```python
from build123d import *

# Parameters (mm, degrees)
EXTRUDE1_DEPTH = 25.146
HOLE1_D        = 16.002
HOLE1_DEPTH    = 2.286
CHAMFER1_SIZE  = 0.254
CHAMFER2_SIZE  = 0.762
CHAMFER3_SIZE  = 0.762
CHAMFER4_SIZE  = 0.762


with BuildPart() as part:
    # Sketch1 → Extrude1 (new body)
    with BuildSketch(Plane(origin=(0, 0, 0), x_dir=(0, -1, 0), z_dir=(-1, 0, 0))):
        Polygon((31.75, 18.330871047), (0, 36.661742094), (-31.75, 18.330871047), (-31.75, -18.330871047), (0, -36.661742094), (31.75, -18.330871047), align=None)
    extrude(amount=-EXTRUDE1_DEPTH)

    # Sketch2 → Cut-Revolve1 (revolve, cut)
    with BuildSketch(Plane.XY, mode=Mode.PRIVATE) as cut_revolve1_sk:
        with BuildLine():
            Line((0, 27.8003), (0, 0))
            Line((0, 0), (25.146, 0))
            Line((25.146, 0), (25.146, 10.4775))
            Line((25.146, 10.4775), (24.892, 10.4775))
            Line((24.892, 10.4775), (24.892, 6.1849))
            Line((24.892, 6.1849), (22.3393, 5.642306865))
            Line((22.3393, 5.642306865), (21.675393135, 4.9784))
            Line((21.675393135, 4.9784), (14.986, 4.9784))
            Line((14.986, 4.9784), (14.986, 27.4955))
            Line((14.986, 27.4955), (12.7, 27.4955))
            ThreePointArc((12.7, 27.4955), (12.512653369, 27.717323293), (12.234410309, 27.8003))
            Line((12.234410309, 27.8003), (0, 27.8003))
        make_face()
    revolve(cut_revolve1_sk.sketch.rotate(Axis((0, 0, 0), (1, 0, 0)), 270), axis=Axis((0, 0, 0), (1, 0, 0)), mode=Mode.SUBTRACT)  # turned: the seam where the file's is

    # Hole1
    with Locations(Plane.ZY.offset(-14.986)):
        with Locations((0, 15.24)):
            Hole(HOLE1_D / 2, depth=HOLE1_DEPTH)

    # Chamfer1
    chamfer1_edges = [part.edges().sort_by_distance(p)[0] for p in [
        (0, 0, 27.8003),
    ]]
    chamfer(chamfer1_edges, length=CHAMFER1_SIZE)

    # Chamfer2
    chamfer2_edges = [part.edges().sort_by_distance(p)[0] for p in [
        (14.986, 0, 4.9784),
    ]]
    chamfer(chamfer2_edges, length=CHAMFER2_SIZE)

    # Chamfer3
    chamfer3_edges = [part.edges().sort_by_distance(p)[0] for p in [
        (0, -15.875, -27.49630657),
        (0, 15.875, -27.49630657),
        (0, 31.75, 0),
        (0, 15.875, 27.49630657),
        (0, -15.875, 27.49630657),
        (0, -31.75, 0),
    ]]
    chamfer(chamfer3_edges, length=CHAMFER3_SIZE)

    # Chamfer4
    chamfer4_edges = [part.edges().sort_by_distance(p)[0] for p in [
        (25.146, 15.875, 27.49630657),
        (25.146, 31.75, 0),
        (25.146, 15.875, -27.49630657),
        (25.146, -15.875, -27.49630657),
        (25.146, -31.75, 0),
        (25.146, -15.875, 27.49630657),
    ]]
    chamfer(chamfer4_edges, length=CHAMFER4_SIZE)


solid = part.part
```
Read the model definition and answer for the solid it produces. Units are mm, in the model's axes. A direction names the side the tool comes from. Coordinates: 2 decimals unless noted, no trailing zeros. Write each loop counter-clockwise with the first axis right and the second up, starting at its lowest first coordinate (ties: lowest second). Pieces come first, ordered by that corner, then holes. Notation, with made-up numbers: (9.5, 87) - (46.5, 87) arc R13 ccw to (46.5, 92) - close; hole circle Ø5 at (48.25, -33.5). An arc over 180 degrees is marked (long way). Answer as a JSON object with one key per item and string values. Group by question number.
1. The mould has two halves that part along Y. Classify faces 4 (the flat face through (24.77, 15.46, 27.29)), 5 (the flat face through (0, 12, -26)), 6 (the flat face through (24.77, -15.46, -27.29)), 7 (the flat face through (14.986, -6, 6)): +Y half, -Y half, draft (parallel to the pull), parting line (faces both ways), or undercut.
2. Each of these flat-tipped pins is pushed along its axis until it touches: P1, Ø8, axis at y = -15.5, z = -17, coming from the -X side; P2, Ø4, axis at x = 5, y = -2.5, coming from the -Z side; P3, Ø1.5, axis at x = 7, z = 20, coming from the +Y side. Where does it stop, or does it pass through?
3. Which of the six approach directions +Z, -Z, +X, -X, +Y, -Y give full straight-line access (tool end or side, diameter ignored) to faces 1 (the flat face through (24.892, -5, -5)), 2 (the flat face through (24.8, 15.9, -27)), 3 (the cylindrical face through (13.83, -26.84, 5.96))?
4. Consider L1, parallel to Y at x = 13.8, z = 0; L2, parallel to X at y = 4, z = 8; L3, parallel to X at y = 11.5, z = 15. Determine where each line is inside the solid, lowest interval first. Write a range as [from, to].
5. A cutting plane is placed at A-A (x = 4.25). Determine the outline of the cut face in (y, z), plus the area to 3 significant figures.
Worked out:
{
 "1": {"face 4": "+Y half", "face 5": "draft", "face 6": "-Y half", "face 7": "undercut"},
 "2": {"P1": "stops at x = 14.99", "P2": "stops at z = -36.37", "P3": "stops at y = 30.16"},
 "3": {"face 1": "+X", "face 2": "-Z, +X, +Y", "face 3": "-X"},
 "4": {"L1": "y = [-31.75, -27.5], [27.5, 31.75]", "L2": "x = [14.99, 24.89]", "L3": "x = [14.99, 25.15]"},
 "5": {"outline": "(-31.75, -18.33) - (0, -36.66) - (31.75, -18.33) - (31.75, 18.33) - (0, 36.66) - (-31.75, 18.33) - close; hole circle Ø55.6 at (0, 0)", "area": "1,060 mm²"}
}
